Design review of the part built by this model. Coordinates are the model's own, in mm. A direction names the side the tool comes from. Round coordinates to 2 decimals unless told otherwise and drop trailing zeros. Loops run counter-clockwise (first coordinate to the right, second up) from the corner with the lowest first, then second, coordinate; pieces in that order, holes last. Notation, with made-up numbers: (2.25, 48.25) -> (54.25, 48.25) arc R30 cw to (54.25, 71.25) -> close; hole circle Ø8 at (89, 29). An arc over 180 degrees is marked (long way). Write each question's results on one line, items separated by ' | '. Start each with the question number.
Autodesk Inventor part; units mm, degrees
ref_plane "YZ Plane" through (0, 0, 0) normal (1, 0, 0) x (0, 1, 0)
ref_plane "XZ Plane" through (0, 0, 0) normal (0, 1, 0) x (-1, 0, 0)
ref_plane "XY Plane" through (0, 0, 0) normal (0, 0, 1) x (1, 0, 0)
sketch "Sketch3" plane through (0, 0, 0) normal (0, 0, 1) x (1, 0, 0)
  line L0 (-8.9702, 53.029) -> (-8.9702, 53.0291)
  line L1 (-8.9702, 53.0291) -> (-4.9702, 53.0291)
  line L2 (-4.9702, 53.0291) -> (-4.9702, 55.029)
  line L3 (-4.9702, 55.029) -> (-87.0018, 55.029)
  arc A0 (-87.0018, 55.029) -> (-89.0018, 53.029) centre (-87.0018, 53.029) ccw
  line L4 (-89.0018, 53.029) -> (-89.0018, -53.029)
  arc A1 (-89.0018, -53.029) -> (-87.0018, -55.029) centre (-87.0018, -53.029) ccw
  line L5 (-87.0018, -55.029) -> (-4.9702, -55.029)
  line L6 (-4.9702, -55.029) -> (-4.9702, -53.029)
  line L7 (-4.9702, -53.029) -> (-8.9702, -53.029)
  line L8 (-8.9702, -53.029) -> (-85.0018, -53.029)
  arc A2 (-87.0018, -51.029) -> (-85.0018, -53.029) centre (-85.0018, -51.029) ccw
  line L9 (-87.0018, -51.029) -> (-87.0018, 51.029)
  arc A3 (-85.0018, 53.029) -> (-87.0018, 51.029) centre (-85.0018, 51.029) ccw
  line L10 (-85.0018, 53.029) -> (-8.9702, 53.029)
  line L11 (49.0298, 53.0291) -> (49.0298, 53.029)
  line L12 (49.0298, 53.029) -> (85.0018, 53.029)
  arc A4 (87.0018, 51.029) -> (85.0018, 53.029) centre (85.0018, 51.029) ccw
  line L13 (87.0018, 51.029) -> (87.0018, -51.029)
  arc A5 (85.0018, -53.029) -> (87.0018, -51.029) centre (85.0018, -51.029) ccw
  line L14 (85.0018, -53.029) -> (49.0298, -53.029)
  line L15 (49.0298, -53.029) -> (45.0298, -53.029)
  line L16 (45.0298, -53.029) -> (45.0298, -55.029)
  line L17 (45.0298, -55.029) -> (87.0018, -55.029)
  arc A6 (87.0018, -55.029) -> (89.0018, -53.029) centre (87.0018, -53.029) ccw
  line L18 (89.0018, -53.029) -> (89.0018, 53.029)
  arc A7 (89.0018, 53.029) -> (87.0018, 55.029) centre (87.0018, 53.029) ccw
  line L19 (87.0018, 55.029) -> (45.0298, 55.029)
  line L20 (45.0298, 55.029) -> (45.0298, 53.0291)
  line L21 (45.0298, 53.0291) -> (49.0298, 53.0291)
  line L22 (87.0018, 55.029) -> (-87.0018, 55.029)
  line L23 (-89.0018, 53.029) -> (-89.0018, -53.029)
  line L24 (-87.0018, -55.029) -> (87.0018, -55.029)
  line L25 (89.0018, -53.029) -> (89.0018, 53.029)
  line L26 (85.1018, 53.129) -> (-85.1018, 53.129)
  line L27 (-87.1018, 51.129) -> (-87.1018, -51.129)
  line L28 (-85.1018, -53.129) -> (85.1018, -53.129)
  line L29 (87.1018, -51.129) -> (87.1018, 51.129)
  arc A8 (89.0018, 53.029) -> (87.0018, 55.029) centre (87.0018, 53.029) ccw
  arc A9 (87.1018, 51.129) -> (85.1018, 53.129) centre (85.1018, 51.129) ccw
  arc A10 (85.1018, -53.129) -> (87.1018, -51.129) centre (85.1018, -51.129) ccw
  arc A11 (87.0018, -55.029) -> (89.0018, -53.029) centre (87.0018, -53.029) ccw
  arc A12 (-87.1018, -51.129) -> (-85.1018, -53.129) centre (-85.1018, -51.129) ccw
  arc A13 (-89.0018, -53.029) -> (-87.0018, -55.029) centre (-87.0018, -53.029) ccw
  arc A14 (-85.1018, 53.129) -> (-87.1018, 51.129) centre (-85.1018, 51.129) ccw
  arc A15 (-87.0018, 55.029) -> (-89.0018, 53.029) centre (-87.0018, 53.029) ccw
  point P0 (0, 0)
  dimension "d0" = 0.1
  dimension "d1" = 0.1
  dimension "d2" = 0.1
  dimension "d3" = 0.1
  dimension "d4" = 2
extrude "Extrusion1" add sketch "Sketch3" along normal blind 4.2 contours L26 A14 L27 A12 L28 L6 L5 A1 L4 A0 L3 L2 | L2 L22 L20 L26 | L20 L19 A7 L18 A6 L17 L16 L28 A10 L29 A9 L26 | L28 L16 L24 L6
sketch "Sketch4" plane through (0, 0, 4.2) normal (0, 0, 1) x (1, 0, 0)
  line L0 (-87.0018, -55.029) -> (87.0018, -55.029)
  arc A0 (87.0018, -55.029) -> (89.0018, -53.029) centre (87.0018, -53.029) ccw
  line L1 (89.0018, -53.029) -> (89.0018, 53.029)
  arc A1 (89.0018, 53.029) -> (87.0018, 55.029) centre (87.0018, 53.029) ccw
  line L2 (87.0018, 55.029) -> (-87.0018, 55.029)
  arc A2 (-87.0018, 55.029) -> (-89.0018, 53.029) centre (-87.0018, 53.029) ccw
  line L3 (-89.0018, 53.029) -> (-89.0018, -53.029)
  arc A3 (-89.0018, -53.029) -> (-87.0018, -55.029) centre (-87.0018, -53.029) ccw
  line L4 (85.1018, -53.129) -> (-85.1018, -53.129)
  arc A4 (-87.1018, -51.129) -> (-85.1018, -53.129) centre (-85.1018, -51.129) ccw
  line L5 (-87.1018, -51.129) -> (-87.1018, 51.129)
  arc A5 (-85.1018, 53.129) -> (-87.1018, 51.129) centre (-85.1018, 51.129) ccw
  line L6 (-85.1018, 53.129) -> (85.1018, 53.129)
  arc A6 (87.1018, 51.129) -> (85.1018, 53.129) centre (85.1018, 51.129) ccw
  line L7 (87.1018, 51.129) -> (87.1018, -51.129)
  arc A7 (85.1018, -53.129) -> (87.1018, -51.129) centre (85.1018, -51.129) ccw
  point P0 (0, 0)
extrude "Extrusion2" add sketch "Sketch4" along normal blind 4.8 contours A3 L3 A2 L2 A1 L1 A0 L0 | L4 A4 L5 A5 L6 A6 L7 A7
sketch "Sketch5" plane through (0, 0, 9) normal (0, 0, 1) x (1, 0, 0)
  circle A0 centre (83.5122, 49.5394) radius 2
  circle A1 centre (83.5122, -49.5394) radius 2
  circle A2 centre (-83.5122, -49.5394) radius 2
  circle A3 centre (-83.5122, 49.5394) radius 2
  circle A4 centre (83.5122, 49.5394) radius 1.45
  circle A5 centre (83.5122, -49.5394) radius 1.45
  circle A6 centre (-83.5122, -49.5394) radius 1.45
  circle A7 centre (-83.5122, 49.5394) radius 1.45
  point P0 (0, 0)
  dimension "d9" = 2.9
  dimension "d10" = 2.9
  dimension "d11" = 2.9
  dimension "d12" = 2.9
extrude "Extrusion3" cut sketch "Sketch5" against normal blind 10 contours A4 | A5 | A6 | A7
chamfer "Chamfer1" distance 1.3 angle 45 4 edges at (82.0622, 49.5394, 9) (82.0622, -49.5394, 9) (-84.9622, 49.5394, 9) (-84.9622, -49.5394, 9)
properties part number "First_Stage_BoxTop_Print"
1) Insertion check: pin 1 (8 mm diameter, centred on x = -59.5, y = -39, fed in from -Z); pin 2 (4 mm diameter, centred on x = 83.51, y = -49.54, fed in from +Z); pin 3 (4.5 mm diameter, centred on x = -83.51, y = 49.54, fed in from +Z). Each pin has a flat end and moves straight along its axis. Give the tip position at first contact, or say it passes through.
2) To check wall thickness, follow line 1 (X direction, y = -42.5, z = 3.5); line 2 (Y direction, x = 35.5, z = 2.75); line 3 (X direction, y = 50.5, z = 6.75). State the ranges of each line that lie inside material, in increasing order. Write a range as from..to.
3) Take a section at C-C (y = -36.5). Write out the cut boundary in (x, z), plus the area to 3 significant figures.
4) The part is to be moulded in two halves that separate along X. For faces 3 (the face through (1, 53.129, 2)), 4 (the face through (1, 55.029, 4)), 5 (the face through (89.002, -1, 4)), say which applies: +X half, -X half, draft (parallel to the pull), parting line (faces both ways), or undercut.
5) Take a section at A-A (z = 2.5). Write out the cut boundary in (x, y).
6) For faces 1 (the face through (-1, 1, 9)), 2 (the face through (-1, -53.129, 2)), list the 3-axis set-ups (+Z, -Z, +X, -X, +Y, -Y) from which the entire face can be reached by the end or side of a thin tool; tool diameter is ignored.
7) Take a section at B-B (x = -67.5). Write out the cut boundary in (y, z).
Geometry check:
1) pin 1: stops at z = 4.2 | pin 2: stops at z = 8.25 | pin 3: stops at z = 8.5
2) line 1: x = -89..-87.1, 87.1..89 | line 2: y = -55.03..-53.13, 53.13..55.03 | line 3: x = -89..-84.6, -82.43..82.43, 84.6..89
3) outline: (-89, 0) -> (-87.1, 0) -> (-87.1, 4.2) -> (87.1, 4.2) -> (87.1, 0) -> (89, 0) -> (89, 9) -> (-89, 9) -> close | area: 870 mm^2
4) face 3: undercut | face 4: draft | face 5: +X half
5) outline: (-89, -53.03) arc R2 ccw to (-87, -55.03) -> (87, -55.03) arc R2 ccw to (89, -53.03) -> (89, 53.03) arc R2 ccw to (87, 55.03) -> (-87, 55.03) arc R2 ccw to (-89, 53.03) -> close; hole (-87.1, -51.13) arc R2 ccw to (-85.1, -53.13) -> (85.1, -53.13) arc R2 ccw to (87.1, -51.13) -> (87.1, 51.13) arc R2 ccw to (85.1, 53.13) -> (-85.1, 53.13) arc R2 ccw to (-87.1, 51.13) -> close
6) face 1: +Z, +X, -X, +Y, -Y | face 2: -Z
7) outline: (-55.03, 0) -> (-53.13, 0) -> (-53.13, 4.2) -> (53.13, 4.2) -> (53.13, 0) -> (55.03, 0) -> (55.03, 9) -> (-55.03, 9) -> close
